Part model, mm, in its own coordinate system. Give positions to 0.01 mm unless a question says otherwise; leave off trailing zeros. Write each loop counter-clockwise with the first axis right and the second up, starting at its lowest first coordinate (ties: lowest second). Pieces come first, ordered by that corner, then holes. Notation, with made-up numbers: M -35.5,76.25 L -15.5,76.25 A26 ccw -15.5,93.25 Z; hole C 80,-9.75 d6. An arc over 180 degrees is marked long. Use CSV: the item, a comma, the result in double quotes. Start each with the question number.
Item 1: Pin check, flat tips, straight feed: pin 1 (4.5 mm diameter, centred on y = 6.5, z = -132.5, fed in from -X); pin 2 (1 mm diameter, centred on x = 26.5, z = -73.5, fed in from -Y); pin 3 (0.8 mm diameter, centred on y = -0.5, z = -4.5, fed in from +X). Stop position of each tip, or through.
Item 2: Cut at A-A (y = 7.5). List the corners of the cut face in (x, z).
Item 3: Drill centre lines: line 1 (X direction, y = 1.15, z = -8.89); line 2 (Y direction, x = 12.5, z = -94); line 3 (X direction, y = 0.5, z = -115.5). Where is each one in solid material? Low to high. Write a range as [from, to].
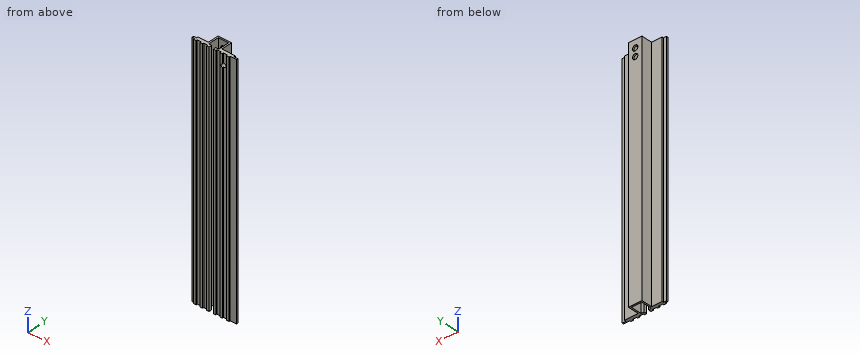
from build123d import *

# Parameters (mm, degrees)
BOSS_EXTRUDE1_DEPTH = 195.58
CUT_EXTRUDE1_REACH  = 201.244
SKETCH2_R           = 2.2225
SKETCH5_R           = 1.524
CUT_EXTRUDE4_DEPTH  = 200.053570631


with BuildPart() as part:
    # Sketch1 → Boss-Extrude1 (new body)
    with BuildSketch(Plane.XY):
        Polygon((0, 0), (2.032, 0), (2.032, -1.016), (4.064, -1.016), (4.064, 0), (7.366, 0), (7.366, -1.016), (9.398, -1.016), (9.398, 0), (12.7, 0), (12.7, -1.016), (14.732, -1.016), (14.732, 0), (14.732, 1.27), (12.192, 1.27), (12.192, 10.16), (20.574, 10.16), (20.574, 1.27), (18.034, 1.27), (18.034, 0), (18.034, -1.016), (20.066, -1.016), (20.066, 0), (23.368, 0), (23.368, -1.016), (25.4, -1.016), (25.4, 0), (28.702, 0), (28.702, -1.016), (30.734, -1.016), (30.734, 0), (32.766, 0), (35.941, 0), (35.941, 1.27), (32.766, 1.27), (32.766, 2.54), (30.226, 2.54), (21.844, 2.54), (21.844, 11.43), (10.922, 11.43), (10.922, 2.54), (2.54, 2.54), (2.54, 1.27), (0, 1.27), align=None)
    extrude(amount=-BOSS_EXTRUDE1_DEPTH)

    # Sketch2 → Cut-Extrude1 (cut, up to next)
    with BuildSketch(Plane(origin=(0, 11.43, 0), x_dir=(1, 0, 0), z_dir=(0, 1, 0)), mode=Mode.PRIVATE) as cut_extrude1_sk1:
        with Locations(Location((16.383, 6.35, 0), (0, 0, 270))):
            Circle(SKETCH2_R)
    cut_extrude1_tool1 = extrude(cut_extrude1_sk1.sketch, amount=-CUT_EXTRUDE1_REACH, mode=Mode.PRIVATE) & part.part
    # Sketch2 → Cut-Extrude1 (cut, up to next)
    with BuildSketch(Plane(origin=(0, 11.43, 0), x_dir=(1, 0, 0), z_dir=(0, 1, 0)), mode=Mode.PRIVATE) as cut_extrude1_sk2:
        with Locations(Location((16.383, 12.7, 0), (0, 0, 270))):
            Circle(SKETCH2_R)
    cut_extrude1_tool2 = extrude(cut_extrude1_sk2.sketch, amount=-CUT_EXTRUDE1_REACH, mode=Mode.PRIVATE) & part.part
    add(cut_extrude1_tool1.solids().sort_by_distance((16.383, 11.43, -6.35))[0], mode=Mode.SUBTRACT)
    add(cut_extrude1_tool2.solids().sort_by_distance((16.383, 11.43, -12.7))[0], mode=Mode.SUBTRACT)

    # Sketch5 → Cut-Extrude4 (cut, through all)
    with BuildSketch(Plane(origin=(0, 2.54, 0), x_dir=(1, 0, 0), z_dir=(0, 1, 0))):
        with Locations(Location((25.908, 8.89, 0), (0, 0, 180))):
            Circle(SKETCH5_R)
    extrude(amount=-CUT_EXTRUDE4_DEPTH, mode=Mode.SUBTRACT)


solid = part.part
Worked answers:
1,pin 1,"stops at x = 10.92"
1,pin 2,"stops at y = 0"
1,pin 3,"stops at x = 30.73"
2,outline,"M 10.92,-195.58 L 12.19,-195.58 L 12.19,0 L 10.92,0 Z; M 20.57,-195.58 L 21.84,-195.58 L 21.84,0 L 20.57,0 Z"
3,line 1,"x = [0, 14.73], [18.03, 24.38], [27.43, 35.94]"
3,line 2,"y = [0, 1.27], [10.16, 11.43]"
3,line 3,"x = [0, 14.73], [18.03, 35.94]"
